```python
from build123d import *

# Parameters (mm, degrees)
SKETCH_1_W             = 80
SKETCH_1_H             = 100
EXTRUDE_1_DEPTH        = 10
HOLE_WIZARD_1_D        = 10
HOLE_WIZARD_M4_1_D     = 3.3
HOLE_WIZARD_M6_1_D     = 5
HOLE_WIZARD_M5_1_D     = 4.2
HOLE_WIZARD_M5_1_DEPTH = 12.4
HOLE_WIZARD_M5_1_TIP   = 1.2618073
HOLE_WIZARD_M5_2_D     = 4.2
HOLE_WIZARD_M5_2_DEPTH = 12.4
HOLE_WIZARD_M5_2_TIP   = 1.2618073
HOLE_WIZARD_M5_3_D     = 4.2
HOLE_WIZARD_M5_3_DEPTH = 10.4
HOLE_WIZARD_M5_3_TIP   = 1.2618073


with BuildPart() as part:
    # 草图1 → 凸台-拉伸1 (new body)
    with BuildSketch(Plane(origin=(0, 0, 0), x_dir=(1, 0, 0), z_dir=(0, 1, 0))):
        Rectangle(SKETCH_1_W, SKETCH_1_H)
    extrude(amount=EXTRUDE_1_DEPTH)

    # 孔1 (through all)
    with Locations(Plane(origin=(0, 10, 0), x_dir=(1, 0, 0), z_dir=(0, 1, 0))):
        with Locations((0, 40)):
            Hole(HOLE_WIZARD_1_D / 2)

    # M4 螺纹孔1 (through all)
    with Locations(Plane(origin=(0, 0, 0), x_dir=(-1, 0, 0), z_dir=(0, -1, 0))):
        with Locations((35, -35), (-35, -35), (-35, 35), (35, 35)):
            Hole(HOLE_WIZARD_M4_1_D / 2)

    # M6 螺纹孔1 (through all)
    with Locations(Plane(origin=(0, 10, 0), x_dir=(1, 0, 0), z_dir=(0, 1, 0))):
        with Locations((-29.071712183, -39.873872767), (29.071712183, -39.873872767)):
            Hole(HOLE_WIZARD_M6_1_D / 2)

    # M5 螺纹孔1
    with Locations(Plane(origin=(40, 0, 0), x_dir=(0, 0, -1), z_dir=(1, 0, 0))):
        with Locations((-17, 5), (-2, 5)):
            Hole(HOLE_WIZARD_M5_1_D / 2, depth=HOLE_WIZARD_M5_1_DEPTH)
            with Locations((0, 0, -(HOLE_WIZARD_M5_1_DEPTH + HOLE_WIZARD_M5_1_TIP / 2))):  # 118° drill point
                Cone(0, HOLE_WIZARD_M5_1_D / 2, HOLE_WIZARD_M5_1_TIP, mode=Mode.SUBTRACT)

    # M5 螺纹孔2
    with Locations(Plane.ZY.offset(40)):
        with Locations((5, 5), (-8, 5)):
            Hole(HOLE_WIZARD_M5_2_D / 2, depth=HOLE_WIZARD_M5_2_DEPTH)
            with Locations((0, 0, -(HOLE_WIZARD_M5_2_DEPTH + HOLE_WIZARD_M5_2_TIP / 2))):  # 118° drill point
                Cone(0, HOLE_WIZARD_M5_2_D / 2, HOLE_WIZARD_M5_2_TIP, mode=Mode.SUBTRACT)

    # M5 螺纹孔3
    with Locations(Plane.XY.offset(50)):
        with Locations((-7.5, 5), (7.5, 5)):
            Hole(HOLE_WIZARD_M5_3_D / 2, depth=HOLE_WIZARD_M5_3_DEPTH)
            with Locations((0, 0, -(HOLE_WIZARD_M5_3_DEPTH + HOLE_WIZARD_M5_3_TIP / 2))):  # 118° drill point
                Cone(0, HOLE_WIZARD_M5_3_D / 2, HOLE_WIZARD_M5_3_TIP, mode=Mode.SUBTRACT)


solid = part.part
```
Build history of the part. All positions in model axes, mm. A direction names the side the tool comes from. Give positions to 0.01 mm unless a question says otherwise; leave off trailing zeros. Loops run counter-clockwise (first coordinate to the right, second up) from the corner with the lowest first, then second, coordinate; pieces in that order, holes last.
1) Probe line 1 along X through (y, z) = (6.75, 35); line 2 along X through (y, z) = (5, 45.75); line 3 along Z through (x, y) = (-35, 7.5). List the from-to ranges inside material, lowest first.
Values follow:
line 1: x = -40 to -36.65, -33.35 to 33.35, 36.65 to 40
line 2: x = -40 to -9.6, -5.4 to 5.4, 9.6 to 40
line 3: z = -50 to -36.65, -33.35 to 33.35, 36.65 to 50
2) Band-saw the part on A-A on z = -40. List the corners of the cut face in (x, y), then the cut area to 3 significant figures.
Values follow:
outline: (-40, 0) - (-5, 0) - (-5, 10) - (-40, 10) - close; (5, 0) - (40, 0) - (40, 10) - (5, 10) - close
area: 700 mm2
3) 3-axis set-ups, long thin cutter, end or side, ignore diameter. For faces 1 (the face through (33.713, 5.631, 19.003)), 2 (the face through (-5.952, 6.419, 44.727)), 3 (the face through (-1, 0, -1)): which of +Z, -Z, +X, -X, +Y, -Y reach the whole face in a straight line?
Values follow:
face 1: +X
face 2: +Z
face 3: +Z, -Z, +X, -X, -Y
4) Band-saw the part on B-B on x = 0. List the corners of the cut face in (y, z), then the cut area to 3 significant figures.
Values follow:
outline: (0, -50) - (10, -50) - (10, -45) - (0, -45) - close; (0, -35) - (10, -35) - (10, 50) - (0, 50) - close
area: 900 mm2
5) Two-plate mould, pull along Z, no slides. Class faces 4 (the face through (-26.56, 5.25, -8.27)), 5 (the face through (9.048, 6.419, 44.727)), 6 (the face through (-7.77, 5.25, 38.56)): released by +Z, released by -Z, zero draft, split by the parting line, or undercut.
Values follow:
face 4: undercut
face 5: zero draft
face 6: released by +Z
6) Band-saw the part on C-C on z = 35. List the corners of the cut face in (x, y).
Values follow:
outline: (-40, 0) - (-36.65, 0) - (-36.65, 10) - (-40, 10) - close; (-33.35, 0) - (33.35, 0) - (33.35, 10) - (-33.35, 10) - close; (36.65, 0) - (40, 0) - (40, 10) - (36.65, 10) - close
7) Drop flat-ended pins along their axis: P1, Ø4.5, axis at x = -35, z = 35, coming from the +Y side; P2, Ø2, axis at x = 35, z = 35, coming from the -Y side. Give the stop position or say it passes through.
Values follow:
P1: stops at y = 10
P2: passes through
